Geometry check sheet. Reference: the model listing, model coordinates, mm. Coordinates: 2 decimals unless noted, no trailing zeros. Write each loop counter-clockwise with the first axis right and the second up, starting at its lowest first coordinate (ties: lowest second). Pieces come first, ordered by that corner, then holes. Notation, with made-up numbers: (-17.75, 20) -> (28.25, 20) arc R16 cw to (28.25, 28) -> close; hole circle Ø11 at (63.5, 88). An arc over 180 degrees is marked (long way). One line per question, with ' | ' between items.
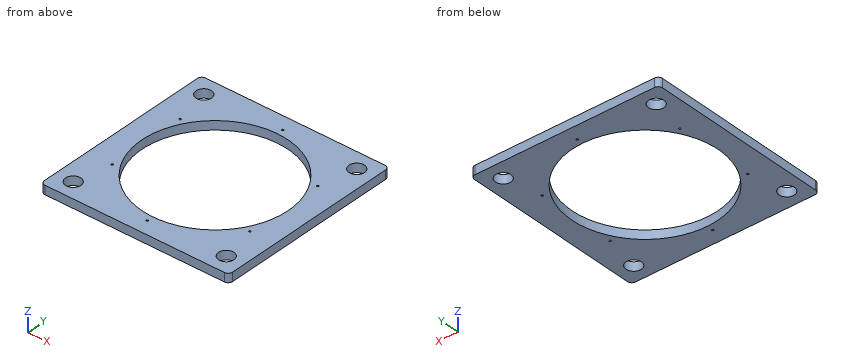
from build123d import *

# Parameters (mm, degrees)
F0_W     = 271.78
F0_H     = 271.78
F1_DEPTH = 12.7
F2_R     = 6.35
F3_R     = 105.41
F4_DEPTH = 25.4
F5_R     = 1.389063
F6_DEPTH = 25.4
F7_R     = 11.1125
F8_DEPTH = 25.4


with BuildPart() as f1:
    # F0 (on Top) → F1 (new body)
    with BuildSketch(Plane.XY):
        Rectangle(F0_W, F0_H)
    extrude(amount=F1_DEPTH)

    # F2
    f2_edges = [f1.edges().sort_by_distance(p)[0] for p in [
        (-135.89, -135.89, 6.35),
        (135.89, -135.89, 6.35),
        (-135.89, 135.89, 6.35),
        (135.89, 135.89, 6.35),
    ]]
    fillet(f2_edges, radius=F2_R)

    # F3 (on face) → F4 (cut)
    with BuildSketch(Plane.XY.offset(12.7)):
        Circle(F3_R)
    extrude(amount=-F4_DEPTH, mode=Mode.SUBTRACT)

    # F5 (on face) → F6 (cut)
    with BuildSketch(Plane.XY.offset(12.7)):
        with Locations((0, 114.808)):
            Circle(F5_R)
        with Locations((99.426645, 57.404)):
            Circle(F5_R)
        with Locations((99.426645, -57.404)):
            Circle(F5_R)
        with Locations((0, -114.808)):
            Circle(F5_R)
        with Locations((-99.426645, -57.404)):
            Circle(F5_R)
        with Locations((-99.426645, 57.404)):
            Circle(F5_R)
    extrude(amount=-F6_DEPTH, mode=Mode.SUBTRACT)

    # F7 (on face) → F8 (cut)
    with BuildSketch(Plane.XY.offset(12.7)):
        with Locations((-110.49, 110.49)):
            Circle(F7_R)
        with Locations((110.49, 110.49)):
            Circle(F7_R)
        with Locations((110.49, -110.49)):
            Circle(F7_R)
        with Locations((-110.49, -110.49)):
            Circle(F7_R)
    extrude(amount=-F8_DEPTH, mode=Mode.SUBTRACT)


solid = f1.part
1. Cross-section at A-A on x = 110.49. Record the boundary of the cut face in (y, z).
Worked answers:
outline: (-135.89, 0) -> (-121.6, 0) -> (-121.6, 12.7) -> (-135.89, 12.7) -> close; (-99.38, 0) -> (99.38, 0) -> (99.38, 12.7) -> (-99.38, 12.7) -> close; (121.6, 0) -> (135.89, 0) -> (135.89, 12.7) -> (121.6, 12.7) -> close
2. Cross-section at D-D on z = 3.5. Give the number of separate pieces and of enclosed holes in the cut face, and give its area (3 significant figures).
Worked answers:
separate pieces: 1 | enclosed holes: 11 | area: 37,300 mm²
3. Cross-section at B-B on y = -95.5. Record the boundary of the cut face in (x, z).
Worked answers:
outline: (-135.89, 0) -> (-44.62, 0) -> (-44.62, 12.7) -> (-135.89, 12.7) -> close; (44.62, 0) -> (135.89, 0) -> (135.89, 12.7) -> (44.62, 12.7) -> close
4. Go/stop test with a flat-tipped pin: P1, Ø2, axis at x = 99.43, y = 57.4, coming from the +Z side. Record where the tip stops, or that it passes through.
Worked answers:
P1: through
5. Material ranges on line 1 (Y direction, x = -110.49, z = 7.75); line 2 (Y direction, x = 0, z = 6.25); line 3 (X direction, y = 112, z = 5), recorded low to high. Write a range as from..to.
Worked answers:
line 1: -135.89..-121.6, -99.38..99.38, 121.6..135.89 | line 2: -135.89..-116.2, -113.42..-105.41, 105.41..113.42, 116.2..135.89 | line 3: -135.89..-121.5, -99.48..99.48, 121.5..135.89
6. Cross-section at C-C on x = -60.5. Record the boundary of the cut face in (y, z), and give its area (3 significant figures).
Worked answers:
outline: (-135.89, 0) -> (-86.32, 0) -> (-86.32, 12.7) -> (-135.89, 12.7) -> close; (86.32, 0) -> (135.89, 0) -> (135.89, 12.7) -> (86.32, 12.7) -> close | area: 1,260 mm²
